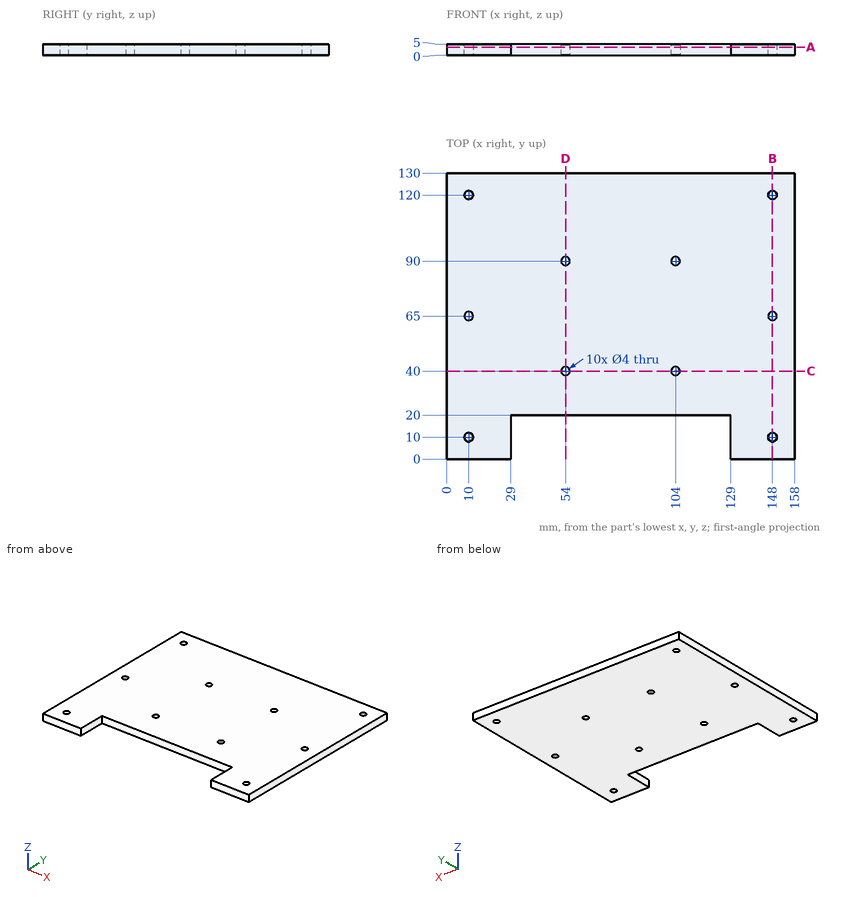
Could you check a few things on this drawing? It's one solid part, dimensions in mm from its lowest x, y, z. Coordinates: 2 decimals unless noted, no trailing zeros. Order: outer loops, then holes, each group sorted by start corner. A loop starts at its lowest first (then second) coordinate and runs counter-clockwise, first axis right, second up. Notation, with made-up numbers: (-7.75, 26.5) - (-2.75, 26.5) arc R20 ccw to (-2.75, 38.5) - close; hole circle Ø4 at (37.25, 28.5). An arc over 180 degrees is marked (long way). One line per question, with ' | ' between items. Start each with the question number.
1. I'm going to push flat-ended pins straight in: pin 1 Ø3 at (x, y) = (104, 90) entering from -Z; pin 2 Ø1.5 at (x, z) = (79.5, 3) entering from -Y. Where does each tip first touch, or does it pass through?
2. If we section it at D-D (x = 54): Write out the boundary of the cut face in (y, z).
3. Please list where these lines run through material, in increasing order: line 1 along X through (y, z) = (120, 1.95); line 2 along Y through (x, z) = (10, 2.75); line 3 along Y through (x, z) = (104, 2.15). Write a range as [from, to].
4. If we section it at C-C (y = 40): Write out the boundary of the cut face in (x, z), and give its area (3 significant figures).
5. If we section it at B-B (x = 148): Write out the boundary of the cut face in (y, z).
6. If we section it at A-A (z = 3.6): Give the number of separate pieces and of enclosed holes in the cut face, and give its area (3 significant figures).
Model answer:
1) pin 1: passes through | pin 2: stops at y = 20
2) outline: (20, 0) - (38, 0) - (38, 5) - (20, 5) - close; (42, 0) - (88, 0) - (88, 5) - (42, 5) - close; (92, 0) - (130, 0) - (130, 5) - (92, 5) - close
3) line 1: x = [0, 8], [12, 146], [150, 158] | line 2: y = [0, 8], [12, 63], [67, 118], [122, 130] | line 3: y = [20, 38], [42, 88], [92, 130]
4) outline: (0, 0) - (52, 0) - (52, 5) - (0, 5) - close; (56, 0) - (102, 0) - (102, 5) - (56, 5) - close; (106, 0) - (158, 0) - (158, 5) - (106, 5) - close | area: 750 mm²
5) outline: (0, 0) - (8, 0) - (8, 5) - (0, 5) - close; (12, 0) - (63, 0) - (63, 5) - (12, 5) - close; (67, 0) - (118, 0) - (118, 5) - (67, 5) - close; (122, 0) - (130, 0) - (130, 5) - (122, 5) - close
6) separate pieces: 1 | enclosed holes: 10 | area: 18,400 mm²
